Geometry: see drawing. Coordinates: mm, zero at the bounding-box minimum. A direction names the side the tool comes from. Round coordinates to 2 decimals unless told otherwise and drop trailing zeros. Order: outer loops, then holes, each group sorted by start corner. A loop starts at its lowest first (then second) coordinate and runs counter-clockwise, first axis right, second up. Notation, with made-up numbers: (2, -9) - (49, -9) arc R15 ccw to (49, 1) - close; hole circle Ø7 at (60.25, 59). An arc over 180 degrees is marked (long way). Put each result on its own line as item: value. Start each with the question number.
1) Line query: probe 1 along X at (y, z) = (14, 1.3); probe 2 along Y at (x, z) = (14, 4). Output: solid intervals per line, ascending. Write a range as [from, to].
2) Access query for the marked faces 5 and 6. Directions: +Z, -Z, +X, -X, +Y, -Y. A direction counts if a zero-diameter tool reaches every point of the face in a straight line with its end or side. Return the directions, or none.
3) Contact query for flat-ended pins moving along their axis: P1, Ø1.5, axis at x = 16.5, z = 1, coming from the -Y side; P2, Ø2, axis at x = 10.5, z = 5.5, coming from the +Y side (3 decimals); P3, Ø1, axis at x = 3, z = 2.5, coming from the -Y side. Output: stop coordinate, or through.
4) Section B-B on z = 3.75. Output: boundary loops of the cut face in (x, y), then the cut area to 3 significant figures.
5) Mould query, pull axis Y, two halves, no side actions, for the marked faces 1, 2, 3 and 4. Classes: +Y half, -Y half, draft (parallel to the pull), parting line (faces both ways), or undercut.
6) Section A-A on x = 14. Output: boundary loops of the cut face in (y, z).
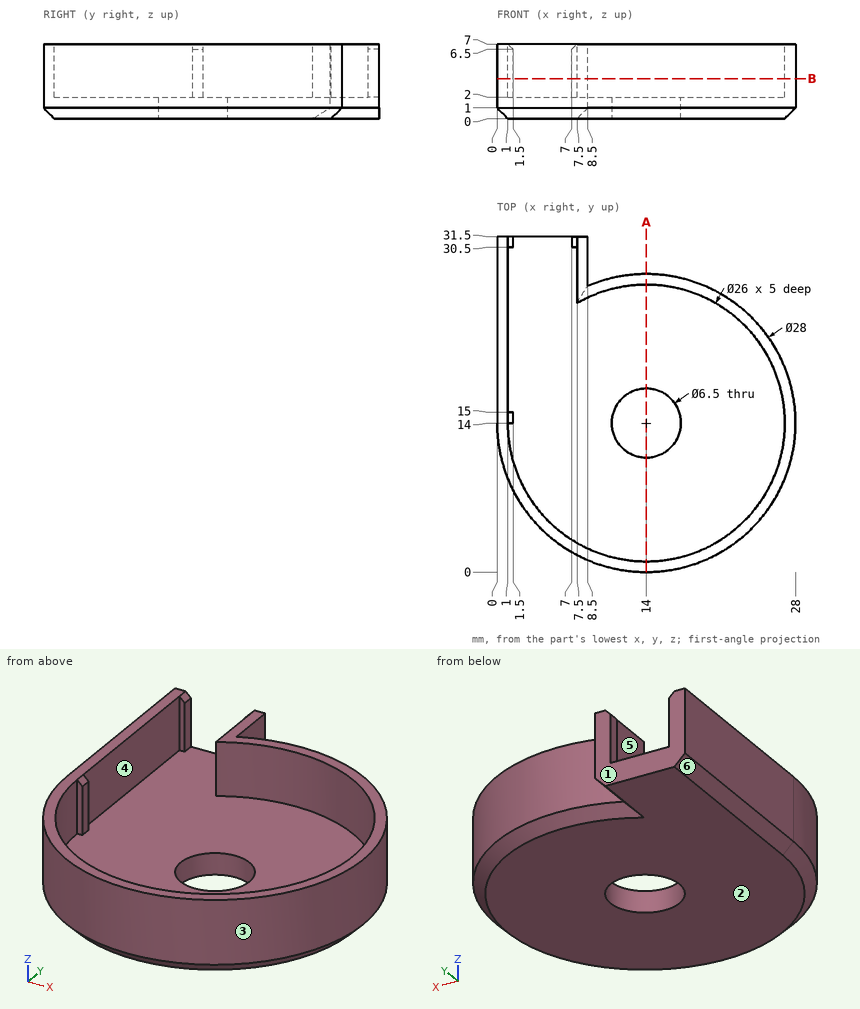
Answer sheet:
1. probe 1: [0, 10.75], [17.25, 28]
1. probe 2: [0, 1], [27, 28]
2. face 5: +Z
2. face 6: -Z, -X, +Y, -Y
3. P1: y = 0.11
3. P2: y = 27.775
3. P3: y = 4.74
4. outline: (0, 14) arc R14 ccw (long way) to (8.5, 26.87) - (8.5, 31.5) - (7, 31.5) - (7, 30.5) - (7.5, 30.5) - (7.5, 25.26) arc R13 cw (long way) to (1, 14) - (1.5, 14) - (1.5, 15) - (1, 15) - (1, 30.5) - (1.5, 30.5) - (1.5, 31.5) - (0, 31.5) - close
4. area: 94.3 mm^2
5. face 1: +Y half
5. face 2: draft
5. face 3: parting line
5. face 4: undercut
6. outline: (0, 1) - (1, 0) - (10.75, 0) - (10.75, 2) - (1, 2) - (1, 7) - (0, 7) - close; (17.25, 0) - (27, 0) - (28, 1) - (28, 7) - (27, 7) - (27, 2) - (17.25, 2) - close
